from build123d import *

# Parameters (mm, degrees)
SKETCH1_W           = 10
SKETCH1_H           = 10
BOSS_EXTRUDE1_DEPTH = 4.2
CUT_EXTRUDE1_REACH  = 10.224
SKETCH3_W           = 0.3
SKETCH3_H           = 2
BOSS_EXTRUDE2_DEPTH = 1.5
SKETCH4_W           = 0.3
SKETCH4_H           = 1
BOSS_EXTRUDE3_DEPTH = 3.7


with BuildPart() as part:
    # Sketch1 → Boss-Extrude1 (new body)
    with BuildSketch(Plane(origin=(0, 0, 0), x_dir=(1, 0, 0), z_dir=(0, 1, 0))):
        Rectangle(SKETCH1_W, SKETCH1_H)
    extrude(amount=-BOSS_EXTRUDE1_DEPTH)

    # Sketch2 → Cut-Extrude1 (cut, up to next)
    with BuildSketch(Plane(origin=(0, 0, 0), x_dir=(1, 0, 0), z_dir=(0, 1, 0)), mode=Mode.PRIVATE) as cut_extrude1_sk1:
        Polygon((1.154700538, 0), (0.577350269, 1), (-0.577350269, 1), (-1.154700538, 0), (-0.577350269, -1), (0.577350269, -1), align=None)
    cut_extrude1_tool1 = extrude(cut_extrude1_sk1.sketch, amount=-CUT_EXTRUDE1_REACH, mode=Mode.PRIVATE) & part.part
    add(cut_extrude1_tool1.solids().sort_by_distance((0, 0, 0))[0], mode=Mode.SUBTRACT)

    # Sketch3 → Boss-Extrude2 (add)
    with BuildSketch(Plane.XZ.offset(4.2)):
        with Locations((4.85, 2.6)):
            Rectangle(SKETCH3_W, SKETCH3_H)
        with Locations((4.85, -2.6)):
            Rectangle(SKETCH3_W, SKETCH3_H)
        with Locations((-4.85, 0)):
            Rectangle(SKETCH3_W, SKETCH3_H)
    extrude(amount=BOSS_EXTRUDE2_DEPTH)

    # Sketch4 → Boss-Extrude3 (add)
    with BuildSketch(Plane.XZ.offset(5.7)):
        with Locations((4.85, -2.6)):
            Rectangle(SKETCH4_W, SKETCH4_H)
        with Locations((-4.85, 0)):
            Rectangle(SKETCH4_W, SKETCH4_H)
        with Locations((4.85, 2.6)):
            Rectangle(SKETCH4_W, SKETCH4_H)
    extrude(amount=BOSS_EXTRUDE3_DEPTH)


solid = part.part
Build history of the part. All positions in model axes, mm. A direction names the side the tool comes from. Give positions to 0.01 mm unless a question says otherwise; leave off trailing zeros. Write each loop counter-clockwise with the first axis right and the second up, starting at its lowest first coordinate (ties: lowest second). Pieces come first, ordered by that corner, then holes. Notation, with made-up numbers: (26, 57) - (39, 57) arc R34 ccw to (39, 89) - close; hole circle Ø9 at (64, -29.5). An arc over 180 degrees is marked (long way). Use one line per item in the form item = value. Start each with the question number.
1. Drop flat-ended pins along their axis: pin 1 Ø2 at (x, y) = (-0.5, -7) entering from +Z; pin 2 Ø1.5 at (x, z) = (2, -0.5) entering from -Y; pin 3 Ø1 at (y, z) = (-6.5, 3) entering from -X. Give the stop position or say it passes through.
2. Band-saw the part on C-C on y = -3.25. Write the cut outline in (x, z).
3. Probe line 1 (Y direction, x = -3.25, z = 2.75); line 2 (Z direction, x = -0.5, y = -2); line 3 (X direction, y = -4.5, z = 2.75). List the from-to ranges inside material, lowest first. Write a range as [from, to].
4. 3-axis set-ups, long thin cutter, end or side, ignore diameter. For faces 1 (the face through (4.7, -6.2, -2.6)), 2 (the face through (-4.7, -6, 0)), 3 (the face through (0.87, -2.07, -0.49)): which of +Z, -Z, +X, -X, +Y, -Y reach the whole face in a straight line?
5. Band-saw the part on D-D on z = 0.25. Write the cut outline in (x, y), plus the area to 3 significant figures.
6. Band-saw the part on B-B on x = -0.25. Write the cut outline in (y, z).
7. Band-saw the part on A-A on y = -4.5. Write the cut outline in (x, z).
8. Two-plate mould, pull along X, no slides. Class faces 4 (the face through (0, -2, -5)), 5 (the face through (4.7, -6.2, 2.6)), 6 (the face through (-0.87, -2.07, 0.49)): released by +X, released by -X, zero draft, split by the parting line, or undercut.
Conclusion:
q1.pin_1 = through
q1.pin_2 = -4.2
q1.pin_3 = 4.7
q2.outline = (-5, -5) - (5, -5) - (5, 5) - (-5, 5) - close; hole (-1.15, 0) - (-0.58, -1) - (0.58, -1) - (1.15, 0) - (0.58, 1) - (-0.58, 1) - close
q3.line_1 = [-4.2, 0]
q3.line_2 = [-5, -1], [1, 5]
q3.line_3 = [4.7, 5]
q4.face_1 = +Z, -Z, -X, -Y
q4.face_2 = +Z, -Z, +X, -Y
q4.face_3 = +Y, -Y
q5.outline = (-5, -9.4) - (-4.7, -9.4) - (-4.7, -4.2) - (-1.01, -4.2) - (-1.01, 0) - (-5, 0) - close; (1.01, -4.2) - (5, -4.2) - (5, 0) - (1.01, 0) - close
q5.area = 35.1 mm²
q6.outline = (-4.2, -5) - (0, -5) - (0, -1) - (-4.2, -1) - close; (-4.2, 1) - (0, 1) - (0, 5) - (-4.2, 5) - close
q7.outline = (-5, -1) - (-4.7, -1) - (-4.7, 1) - (-5, 1) - close; (4.7, -3.6) - (5, -3.6) - (5, -1.6) - (4.7, -1.6) - close; (4.7, 1.6) - (5, 1.6) - (5, 3.6) - (4.7, 3.6) - close
q8.face_4 = zero draft
q8.face_5 = released by -X
q8.face_6 = undercut
